Autodesk Inventor part; units mm, degrees
ref_plane "YZ Plane" through (0, 0, 0) normal (1, 0, 0) x (0, 1, 0)
ref_plane "XZ Plane" through (0, 0, 0) normal (0, 1, 0) x (-1, 0, 0)
ref_plane "XY Plane" through (0, 0, 0) normal (0, 0, 1) x (1, 0, 0)
sketch "Sketch1" plane through (0, 0, 0) normal (0, 0, 1) x (1, 0, 0)
  line L0 (-25.4, -38.1) -> (25.4, -38.1)
  line L1 (25.4, -38.1) -> (25.4, 38.1)
  line L2 (25.4, 38.1) -> (-25.4, 38.1)
  line L3 (-25.4, 38.1) -> (-25.4, -38.1)
  line L4 (-25.4, -38.1) -> (25.4, 38.1) construction
  line L5 (25.4, -38.1) -> (-25.4, 38.1) construction
  line L6 (-22.225, -34.925) -> (22.225, -34.925)
  line L7 (22.225, -34.925) -> (22.225, 34.925)
  line L8 (22.225, 34.925) -> (-22.225, 34.925)
  line L9 (-22.225, 34.925) -> (-22.225, -34.925)
  line L10 (-22.225, -34.925) -> (22.225, 34.925) construction
  line L11 (22.225, -34.925) -> (-22.225, 34.925) construction
  point P0 (0, 0)
  dimension "d0" = 50.8
  dimension "d1" = 76.2
  dimension "d2" = 3.175
  dimension "d3" = 3.175
extrude "Extrusion1" add sketch "Sketch1" against normal blind 304.8
properties part number "2x2x1_8_rectangularTubing" material "Aluminum 6061"
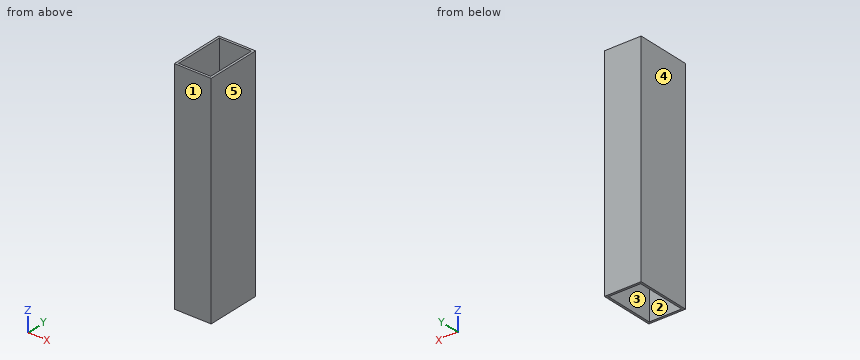
Can you work these out from the model? Positions are in its coordinate system, mm. Face numbers are marked on the shaded views. A direction names the side the tool comes from. Give positions to 0.01 mm unless a question says otherwise; leave off trailing zeros. Write each loop counter-clockwise with the first axis right and the second up, starting at its lowest first coordinate (ties: lowest second). Pieces come first, ordered by that corner, then holes. Notation, with made-up numbers: (-10, -7) - (44, -7) arc R22 ccw to (44, 5) - close; hole circle Ø2 at (-9, 23.25). An arc over 180 degrees is marked (long way). Write item = value, one per line. Start each with the question number.
1. On a 3-axis mill with a long thin cutter (end or side, diameter ignored), from which of +Z, -Z, +X, -X, +Y, -Y can I reach the whole of each face in a straight line? I mean the marked faces 1 and 2. Say none if no direction works.
2. Please list where these lines run through material, in increasing order: line 1 (Y direction, x = 15, z = -285) (3 decimals); line 2 (X direction, y = -29, z = -149.5) (3 decimals).
3. Thinking about a two-plate mould opening in X: for the marked faces 3, 4 and 5, which applies, released by +X, released by -X, zero draft, split by the parting line, or undercut?
4. Imagine slicing it at B-B (y = -24). Please give me the cut outline in (x, z) (3 decimals), and give its area (3 significant figures).
5. Imagine slicing it at C-C (z = -120). Please give me the cut outline in (x, y) (3 decimals).
6. Imagine slicing it at A-A (x = 17). Please give me the cut outline in (y, z) (3 decimals), and give its area (3 significant figures).
Worked answers:
q1.face_1 = +Z, -Z, +X, -X, -Y
q1.face_2 = +Z, -Z
q2.line_1 = -38.1 to -34.925, 34.925 to 38.1
q2.line_2 = -25.4 to -22.225, 22.225 to 25.4
q3.face_3 = undercut
q3.face_4 = released by -X
q3.face_5 = released by +X
q4.outline = (-25.4, -304.8) - (-22.225, -304.8) - (-22.225, 0) - (-25.4, 0) - close; (22.225, -304.8) - (25.4, -304.8) - (25.4, 0) - (22.225, 0) - close
q4.area = 1,940 mm2
q5.outline = (-25.4, -38.1) - (25.4, -38.1) - (25.4, 38.1) - (-25.4, 38.1) - close; hole (-22.225, -34.925) - (22.225, -34.925) - (22.225, 34.925) - (-22.225, 34.925) - close
q6.outline = (-38.1, -304.8) - (-34.925, -304.8) - (-34.925, 0) - (-38.1, 0) - close; (34.925, -304.8) - (38.1, -304.8) - (38.1, 0) - (34.925, 0) - close
q6.area = 1,940 mm2
